from build123d import *

# Parameters (mm, degrees)
SKETCH_W          = 62
SKETCH_H          = 24
PAD_DEPTH         = 62
SKETCH001_W       = 58
SKETCH001_H       = 20
POCKET_DEPTH      = 60
SKETCH002_W       = 8
SKETCH002_H       = 12
POCKET001_DEPTH   = 2
POCKET001_FACE5_W = 24
POCKET001_FACE5_H = 62
PAD001_DEPTH      = 74
PAD001_FACE12_W   = 24
PAD001_FACE12_H   = 74
PAD002_DEPTH      = 74
PAD002_FACE18_W   = 24
PAD002_FACE18_H   = 62
PAD003_DEPTH      = 2
PAD003_FACE24_W   = 24
PAD003_FACE24_H   = 74
PAD004_DEPTH      = 2
SKETCH003_W       = 72
SKETCH003_H       = 16
POCKET002_DEPTH   = 135
FILLET_R          = 3
FILLET001_R       = 3
FILLET002_R       = 3
FILLET003_R       = 3
FILLET004_R       = 1.5
FILLET005_R       = 1.5
FILLET006_R       = 1.5


with BuildPart() as part:
    # Sketch → Pad (new body)
    with BuildSketch(Plane.XY):
        with Locations((31, 12)):
            Rectangle(SKETCH_W, SKETCH_H)
    extrude(amount=PAD_DEPTH)

    # Sketch001 (on Face6 of Pad) → Pocket (cut)
    with BuildSketch(Plane.XY.offset(62)):
        with Locations((31, 12)):
            Rectangle(SKETCH001_W, SKETCH001_H)
    extrude(amount=-POCKET_DEPTH, mode=Mode.SUBTRACT)

    # Sketch002 (on Face1 of Pocket) → Pocket001 (cut)
    with BuildSketch(Plane.XZ):
        with Locations((49, 48)):
            Rectangle(SKETCH002_W, SKETCH002_H)
    extrude(amount=-POCKET001_DEPTH, mode=Mode.SUBTRACT)

    # Pocket001 Face5 → Pad001 (add)
    with BuildSketch(Plane(origin=(62, 12, 31), x_dir=(0, -1, 0), z_dir=(1, 0, 0))):
        Rectangle(POCKET001_FACE5_W, POCKET001_FACE5_H)
    extrude(amount=PAD001_DEPTH)

    # Pad001 Face12 → Pad002 (add)
    with BuildSketch(Plane(origin=(99, 12, 62), x_dir=(0, 1, 0), z_dir=(0, 0, 1))):
        Rectangle(PAD001_FACE12_W, PAD001_FACE12_H)
    extrude(amount=PAD002_DEPTH)

    # Pad002 Face18 → Pad003 (add)
    with BuildSketch(Plane(origin=(136, 12, 31), x_dir=(0, -1, 0), z_dir=(1, 0, 0))):
        Rectangle(PAD002_FACE18_W, PAD002_FACE18_H)
    extrude(amount=PAD003_DEPTH)

    # Pad003 Face24 → Pad004 (add)
    with BuildSketch(Plane(origin=(136, 12, 99), x_dir=(0, -1, 0), z_dir=(1, 0, 0))):
        Rectangle(PAD003_FACE24_W, PAD003_FACE24_H)
    extrude(amount=PAD004_DEPTH)

    # Sketch003 (on Face21 of Pad002) → Pocket002 (cut)
    with BuildSketch(Plane.XY.offset(136)):
        with Locations((100, 12)):
            Rectangle(SKETCH003_W, SKETCH003_H)
    extrude(amount=-POCKET002_DEPTH, mode=Mode.SUBTRACT)

    # Fillet
    fillet_edges = [part.edges().sort_by_distance(p)[0] for p in [
        (45, 1, 42),
    ]]
    fillet(fillet_edges, radius=FILLET_R)

    # Fillet001
    fillet001_edges = [part.edges().sort_by_distance(p)[0] for p in [
        (53, 1, 42),
    ]]
    fillet(fillet001_edges, radius=FILLET001_R)

    # Fillet002
    fillet002_edges = [part.edges().sort_by_distance(p)[0] for p in [
        (53, 1, 54),
    ]]
    fillet(fillet002_edges, radius=FILLET002_R)

    # Fillet003
    fillet003_edges = [part.edges().sort_by_distance(p)[0] for p in [
        (45, 1, 54),
    ]]
    fillet(fillet003_edges, radius=FILLET003_R)

    # Fillet004
    fillet004_edges = [part.edges().sort_by_distance(p)[0] for p in [
        (62, 12, 136),
    ]]
    fillet(fillet004_edges, radius=FILLET004_R)

    # Fillet005
    fillet005_edges = [part.edges().sort_by_distance(p)[0] for p in [
        (138, 12, 136),
    ]]
    fillet(fillet005_edges, radius=FILLET005_R)

    # Fillet006
    fillet006_edges = [part.edges().sort_by_distance(p)[0] for p in [
        (0, 12, 62),
    ]]
    fillet(fillet006_edges, radius=FILLET006_R)


solid = part.part
Source: CAD feature listing. Evaluate the final solid. Frame: model axes, mm. A direction names the side the tool comes from. Give positions to 0.01 mm unless a question says otherwise; leave off trailing zeros. Write each loop counter-clockwise with the first axis right and the second up, starting at its lowest first coordinate (ties: lowest second). Pieces come first, ordered by that corner, then holes. Notation, with made-up numbers: (-2, 46) - (35, 46) arc R7 cw to (35, 53) - close; hole circle Ø5 at (54, 27). An arc over 180 degrees is marked (long way). Write item = value, one per line. Start each with the question number.
Q1. Cut plane B-B, the plane x = 105.5. Return loops of the section in (y, z).
Q2. Pin query (flat end, axial travel): pin 1 Ø2 at (x, y) = (16, 10.5) entering from +Z; pin 2 Ø0.6 at (x, y) = (49, 0.5) entering from +Z; pin 3 Ø1 at (x, y) = (97.5, 13) entering from +Z. Return the tip coordinate at first contact, or that it passes through.
Q3. Material intervals for probe 1 along X at (y, z) = (16.25, 45); probe 2 along Y at (x, z) = (32, 46.5); probe 3 along X at (y, z) = (16.75, 104), sorted ascending.
Q4. Reachability of faces 1 (the flat face through (2, 12, 32)), 2 (the flat face through (38, 23, 62)), 3 (the cylindrical face through (45.86, 1.01, 42.9)) from +Z, -Z, +X, -X, +Y, -Y: full face, straight path, thin tool, end or side. Return the list, or none.
Q5. Cut plane C-C, the plane z = 74. Return loops of the section in (x, y), then the cut area to 3 significant figures.
Q6. Cut plane A-A, the plane z = 29. Return loops of the section in (x, y), then the cut area to 3 significant figures.
Q7. Cut plane D-D, the plane y = 17. Return loops of the section in (x, z).
Q8. Draft query along Z for faces 4 (the cylindrical face through (52.14, 1.01, 53.1)), 5 (the flat face through (99, 20, 69)), 6 (the flat face through (97, 21, 136)). Return one class per face: +Z half, -Z half, draft (parallel to the pull), parting line (faces both ways), or undercut.
Computed values:
q1.outline = (0, 0) - (24, 0) - (24, 136) - (20, 136) - (20, 1) - (4, 1) - (4, 136) - (0, 136) - close
q2.pin_1 = 2
q2.pin_2 = 62
q2.pin_3 = 1
q3.probe_1 = 0 to 2, 60 to 64, 136 to 138
q3.probe_2 = 0 to 2, 22 to 24
q3.probe_3 = 62 to 64, 136 to 138
q4.face_1 = +Z
q4.face_2 = +Z, -X, +Y, -Y
q4.face_3 = -Y
q5.outline = (62, 0) - (138, 0) - (138, 24) - (62, 24) - close; hole (64, 4) - (136, 4) - (136, 20) - (64, 20) - close
q5.area = 672 mm²
q6.outline = (0, 0) - (138, 0) - (138, 24) - (0, 24) - close; hole (2, 2) - (60, 2) - (60, 22) - (2, 22) - close; hole (64, 4) - (136, 4) - (136, 20) - (64, 20) - close
q6.area = 1,000 mm²
q7.outline = (0, 0) - (138, 0) - (138, 134.5) arc R1.5 ccw to (136.5, 136) - (136, 136) - (136, 1) - (64, 1) - (64, 136) - (63.5, 136) arc R1.5 ccw to (62, 134.5) - (62, 62) - (60, 62) - (60, 2) - (2, 2) - (2, 62) - (1.5, 62) arc R1.5 ccw to (0, 60.5) - close
q8.face_4 = undercut
q8.face_5 = draft
q8.face_6 = +Z half
